Could you check a few things on this model? Use its own coordinates, in mm. Face numbers are marked on the shaded views. A direction names the side the tool comes from. Round coordinates to 2 decimals unless told otherwise and drop trailing zeros. Loops run counter-clockwise (first coordinate to the right, second up) from the corner with the lowest first, then second, coordinate; pieces in that order, holes last. Notation, with made-up numbers: (62.5, 62) - (110.5, 62) arc R26 cw to (110.5, 97) - close; hole circle Ø11 at (-39.75, 54). An arc over 180 degrees is marked (long way). Answer as CSV lines item,"result". Start each with the question number.
1) I'm going to push flat-ended pins straight in: pin 1 Ø5 at (y, z) = (8.5, 21.5) entering from -X; pin 2 Ø1.5 at (y, z) = (20.5, 24) entering from +X; pin 3 Ø6 at (x, y) = (10.5, 23) entering from +Z. Where does each tip first touch, or does it pass through?
2) Suppose I cut it at B-B, the plane x = 19.75. Write out the boundary of the cut face in (y, z), then the cut area to 3 significant figures.
3) Suppose I cut it at D-D, the plane x = 13.25. Write out the boundary of the cut face in (y, z).
4) Please list where these lines run through material, in increasing order: line 1 along Z through (x, y) = (5.5, 26.5); line 2 along Y through (x, z) = (11, 18.5); line 3 along X through (y, z) = (14, 15.5).
5) Which directions (+Z, -Z, +X, -X, +Y, -Y) give clear straight access to the entire face, cutting with the end or side of a thin tool? Please do the marked faces 1, 2, 3 and 4.
6) Suppose I cut it at C-C, the plane z = 10.25. Write out the boundary of the cut face in (x, y), then the cut area to 3 significant figures.
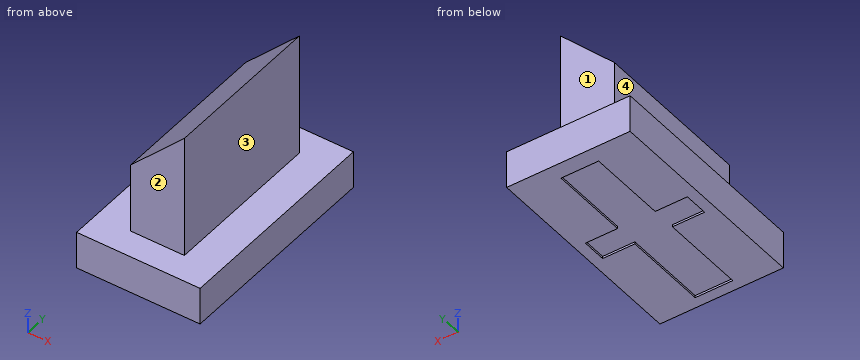
```python
from build123d import *

# Parameters (mm, degrees)
F0_W     = 23
F0_H     = 40
F1_DEPTH = 7
F2_W     = 10
F2_H     = 30
F3_DEPTH = 30
F5_DEPTH = 0.4
F6_SIZE  = 9.99999


# Not quite as in the source:
# - a fillet or chamfer is up to 0.001 mm smaller than in the source, because OpenCascade refuses the exact size


with BuildPart() as f1:
    # F0 (on Top) → F1 (new body)
    with BuildSketch(Plane.XY):
        with Locations((11.5, 20)):
            Rectangle(F0_W, F0_H)
    extrude(amount=F1_DEPTH)

    # F2 (on Top) → F3 (join)
    with BuildSketch(Plane.XY):
        with Locations((11.5, 20)):
            Rectangle(F2_W, F2_H)
    extrude(amount=F3_DEPTH)

    # F4 (on Top) → F5 (cut)
    with BuildSketch(Plane.XY):
        Polygon((8, 17.75), (8, 2), (15, 2), (15, 17.75), (21, 17.75), (21, 22.25), (15, 22.25), (15, 37), (8, 37), (8, 22.25), (2, 22.25), (2, 17.75), align=None)
    extrude(amount=F5_DEPTH, mode=Mode.SUBTRACT)

    # F6 (size 10 in the source; OpenCascade refuses exactly that, so slightly less here)
    f6_edges = [f1.edges().sort_by_distance(p)[0] for p in [
        (6.5, 20, 30),
    ]]
    chamfer(f6_edges, length=F6_SIZE)


solid = f1.part
```
Filled sheet:
1,pin 1,"x = 6.5"
1,pin 2,"x = 16.5"
1,pin 3,"z = 27"
2,outline,"(0, 0) - (17.75, 0) - (17.75, 0.4) - (22.25, 0.4) - (22.25, 0) - (40, 0) - (40, 7) - (0, 7) - close"
2,area,"278 mm²"
3,outline,"(0, 0) - (2, 0) - (2, 0.4) - (37, 0.4) - (37, 0) - (40, 0) - (40, 7) - (35, 7) - (35, 26.75) - (5, 26.75) - (5, 7) - (0, 7) - close"
4,line 1,"0 to 7"
4,line 2,"5 to 35"
4,line 3,"6.5 to 16.5"
5,face 1,"+Z, +X, -X, +Y"
5,face 2,"+Z, +X, -X, -Y"
5,face 3,"+Z, +X, +Y, -Y"
5,face 4,"+Z, -X, +Y, -Y"
6,outline,"(6.5, 5) - (16.5, 5) - (16.5, 35) - (6.5, 35) - close"
6,area,"300 mm²"
